The listing builds one solid part. Answer for the finished solid, in the listing's coordinates (mm). Face numbers are marked on the shaded views. Coordinates: 2 decimals unless noted, no trailing zeros. Order: outer loops, then holes, each group sorted by start corner. A loop starts at its lowest first (then second) coordinate and runs counter-clockwise, first axis right, second up. Notation, with made-up numbers: (61, -32.5) - (78, -32.5) arc R16 cw to (78, -28.5) - close; hole circle Ø3 at (23, -33). An arc over 180 degrees is marked (long way). Use a Markdown table: item, result. Add a question column.
Item 1: Flat-ended cylindrical pins translate along their axes: P1, Ø2, axis at y = 2, z = 6.5, coming from the -X side; P2, Ø2, axis at x = 3, z = 5.5, coming from the -Y side; P3, Ø5, axis at y = -3, z = 7.5, coming from the +X side. Find the tip coordinate at first contact, or state that the pin passes through.
Item 2: The mould has two halves that part along Z. Classify the marked faces 1, 2 and 3: released by +Z, released by -Z, zero draft, split by the parting line, or undercut.
Item 3: The part is cut by section D-D, the plane z = 4.75. Give the vertices of the cut face in (x, y), then the cut area to 3 significant figures.
Item 4: The part is cut by section C-C, the plane x = 0.75. State how many separate pieces and enclosed holes the cut face has, then the cut area to 3 significant figures.
Item 5: The part is cut by section A-A, the plane y = 0. Give the vertices of the cut face in (x, z) (3 decimals), then the cut area to 3 significant figures.
Item 6: The part is cut by section B-B, the plane z = 6. Give the vertices of the cut face in (x, y), then the cut area to 3 significant figures.
Item 7: Find the intervals of material crossed by line 1 along Z through (x, y) = (0, 3.35); line 2 along X through (y, z) = (2.7, 3.4); line 3 along X through (y, z) = (3.6, 3.4), in increasing order.
from build123d import *

# Parameters (mm, degrees)
F0_R     = 4.5
F0_R_2   = 2.25
F1_DEPTH = 11
F2_R     = 1.5
F3_DEPTH = 4.501
F2_R_2   = 2


with BuildPart() as f1:
    # F0 (on Top) → F1 (new body)
    with BuildSketch(Plane.XY):
        Circle(F0_R)
        Circle(F0_R_2, mode=Mode.SUBTRACT)
    extrude(amount=F1_DEPTH)

    # F2 (on Front) → F3 (cut, through all)
    with BuildSketch(Plane.XZ):
        with Locations((0, 3.4)):
            Circle(F2_R)
    extrude(amount=-F3_DEPTH, mode=Mode.SUBTRACT)

    # F2 (on Front) → F4 (revolve, cut)
    with BuildSketch(Plane.XZ):
        with Locations((-5.475, 8)):
            Circle(F2_R_2)
    revolve(axis=Axis((0, 0, 6.367243), (0, 0, -1)), mode=Mode.SUBTRACT)


solid = f1.part
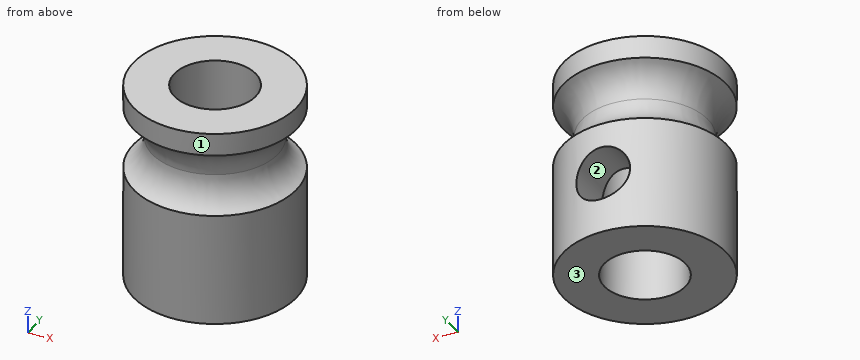
Solution:
| question | item | result |
|---|---|---|
| 1 | P1 | stops at x = -4.38 |
| 1 | P2 | stops at y = -4.03 |
| 1 | P3 | stops at x = 4.42 |
| 2 | face 1 | zero draft |
| 2 | face 2 | undercut |
| 2 | face 3 | released by -Z |
| 3 | outline | (-0.65, 2.15) - (-0.65, 4.45) arc R4.5 ccw (long way) to (0.65, 4.45) - (0.65, 2.15) arc R2.25 cw (long way) to start |
| 3 | area | 44.7 mm2 |
| 4 | separate pieces | 3 |
| 4 | enclosed holes | 0 |
| 4 | area | 39.8 mm2 |
| 5 | outline | (-4.5, 0) - (-2.25, 0) - (-2.25, 11) - (-4.5, 11) - (-4.5, 9.746) arc R2 cw to (-4.5, 6.254) - close; (2.25, 0) - (4.5, 0) - (4.5, 6.254) arc R2 cw to (4.5, 9.746) - (4.5, 11) - (2.25, 11) - close |
| 5 | area | 44.4 mm2 |
| 6 | outline | circle Ø9 at (0, 0); hole circle Ø4.5 at (0, 0) |
| 6 | area | 47.7 mm2 |
| 7 | line 1 | z = 0 to 1.9, 4.9 to 11 |
| 7 | line 2 | x = -3.6 to -1.5, 1.5 to 3.6 |
| 7 | line 3 | x = -2.7 to -1.5, 1.5 to 2.7 |
